```python
from build123d import *

# Parameters (mm, degrees)
SKETCH_R        = 15
PAD_DEPTH       = 7
SKETCH001_R     = 13
POCKET_DEPTH    = 6
SKETCH002_W     = 4.722303
SKETCH002_H     = 6
POCKET001_DEPTH = 6
SKETCH003_R     = 5
POCKET002_DEPTH = 1.001


with BuildPart() as part:
    # Sketch → Pad (new body)
    with BuildSketch(Plane.XY):
        Circle(SKETCH_R)
    extrude(amount=PAD_DEPTH)

    # Sketch001 (on Face3 of Pad) → Pocket (cut)
    with BuildSketch(Plane.XY.offset(7)):
        Circle(SKETCH001_R)
    extrude(amount=-POCKET_DEPTH, mode=Mode.SUBTRACT)

    # Sketch002 (on Face3 of Pocket) → Pocket001 (cut)
    with BuildSketch(Plane.XY.offset(7)):
        with Locations((-13.693224, 3)):
            Rectangle(SKETCH002_W, SKETCH002_H)
    extrude(amount=-POCKET001_DEPTH, mode=Mode.SUBTRACT)

    # Sketch003 (on Face10 of Pocket001) → Pocket002 (cut, through all)
    with BuildSketch(Plane.XY.offset(1)):
        Circle(SKETCH003_R)
    extrude(amount=-POCKET002_DEPTH, mode=Mode.SUBTRACT)


solid = part.part
```
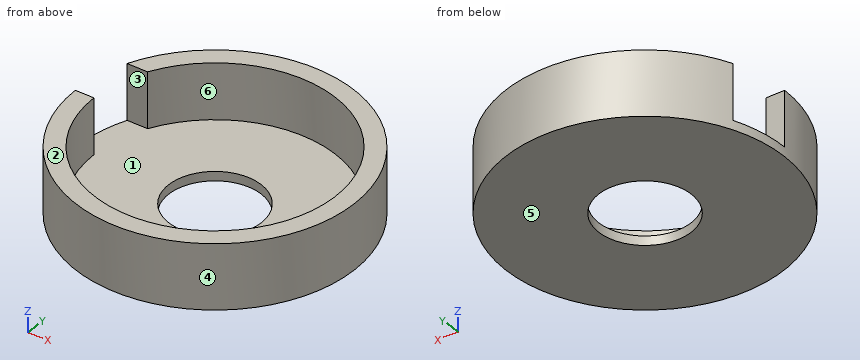
Check sheet for the modelled part. Datum: model origin and axes. Units: mm. Face numbers are marked on the shaded views. A direction names the side the tool comes from. Round coordinates to 2 decimals unless told otherwise and drop trailing zeros. Write each loop counter-clockwise with the first axis right and the second up, starting at its lowest first coordinate (ties: lowest second). Pieces come first, ordered by that corner, then holes. Notation, with made-up numbers: M 79.5,13 L 97.5,13 A22 cw 97.5,44 Z; hole C 31.5,-3 d11. An arc over 180 degrees is marked long. Write item = value, one per line. Start each with the question number.
1. Section check A-A, the plane x = 0. Record the cut outline in (y, z), then the cut area to 3 significant figures.
2. Section check B-B, the plane z = 4.75. Record the cut outline in (x, y), then the cut area to 3 significant figures.
3. Scan lines: line 1 (Y direction, x = 0, z = 2.85); line 2 (Y direction, x = 0, z = 0.45); line 3 (Z direction, x = 1, y = 8.5). Record each from-to range of solid material in increasing order. Write a range as [from, to].
4. Tool access check on the marked faces 1, 2 and 3. Record the directions out of +Z, -Z, +X, -X, +Y, -Y that give a thin tool (end or side, any length) a straight path to the whole face; none if there is none.
5. Gauge pin test, flat ends, axial feed: pin 1 (1.6 mm diameter, centred on x = -13.5, z = 5.5, fed in from +Y); pin 2 (3 mm diameter, centred on x = 2.5, z = 6, fed in from +Y); pin 3 (1 mm diameter, centred on x = 3.5, z = 4, fed in from +Y); pin 4 (12 mm diameter, centred on x = 1, y = -12, fed in from +Z). Record the tip position at first contact, or that the pin passes through.
6. Section check D-D, the plane x = 11. Record the cut outline in (y, z), then the cut area to 3 significant figures.
7. Release check for a two-part mould opening along X. For the marked faces 4, 5 and 6 record: pulls with the +X half, pulls with the -X half, needs draft (parallel to the pull), parting line crosses it, or undercut.
8. Section check C-C, the plane y = 6.5. Record the cut outline in (x, z), then the cut area to 3 significant figures.
Results found:
q1.outline = M -15,0 L -5,0 L -5,1 L -13,1 L -13,7 L -15,7 Z; M 5,0 L 15,0 L 15,7 L 13,7 L 13,1 L 5,1 Z
q1.area = 44.0 mm^2
q2.outline = M -15,0 A15 ccw long -13.75,6 L -11.53,6 A13 cw long -13,0 Z
q2.area = 164 mm^2
q3.line_1 = [-15, -13], [13, 15]
q3.line_2 = [-15, -5], [5, 15]
q3.line_3 = [0, 1]
q4.face_1 = +Z
q4.face_2 = +Z, +X, -X, +Y, -Y
q4.face_3 = +Z, -X
q5.pin_1 = 7.98
q5.pin_2 = 14.97
q5.pin_3 = 14.7
q5.pin_4 = 7
q6.outline = M -10.2,0 L 10.2,0 L 10.2,7 L 6.93,7 L 6.93,1 L -6.93,1 L -6.93,7 L -10.2,7 Z
q6.area = 59.6 mm^2
q7.face_4 = parting line crosses it
q7.face_5 = needs draft
q7.face_6 = undercut
q8.outline = M -13.52,0 L 13.52,0 L 13.52,7 L 11.26,7 L 11.26,1 L -11.26,1 L -11.26,7 L -13.52,7 Z
q8.area = 54.2 mm^2
